Part model, mm, in its own coordinate system. A direction names the side the tool comes from. Give positions to 0.01 mm unless a question says otherwise; leave off trailing zeros. Write each loop counter-clockwise with the first axis right and the second up, starting at its lowest first coordinate (ties: lowest second). Pieces come first, ordered by that corner, then holes.
from build123d import *

# Parameters (mm, degrees)
SKETCH_1_R          = 1.680805835
SKETCH_1_R_2        = 0.406348663
SKETCH_1_R_3        = 0.591052601
SKETCH_1_R_4        = 0.609522995
SKETCH_1_R_5        = 0.664934176
SKETCH_1_R_6        = 1.662335441
SKETCH_1_R_7        = 1.6
EXTRUDE_2_DEPTH     = 1.5
SKETCH_2_W          = 5
SKETCH_2_H          = 30
EXTRUDE_3_DEPTH     = 5
SKETCH_3_W          = 46
SKETCH_3_H          = 35.259040571
EXTRUDE_4_DEPTH     = 1.2
SKETCH_4_W          = 16.562645757
SKETCH_4_H          = 20.676210758
EXTRUDE_5_DEPTH     = 15
SKETCH_5_W          = 14
SKETCH_5_H          = 12
CUT_EXTRUDE_1_DEPTH = 16
SKETCH_6_W          = 12.857554965
SKETCH_6_H          = 12.912362425
EXTRUDE_6_DEPTH     = 5
SKETCH_9_W          = 3.8
SKETCH_9_H          = 10.912362425
CUT_EXTRUDE_2_DEPTH = 11


with BuildPart() as part:
    # 草图1 → 凸台-拉伸2 (new body)
    with BuildSketch(Plane.XY):
        with BuildLine():
            Line((42.436427683, 56.053220537), (165.136427683, 56.053220537))
            ThreePointArc((165.136427683, 56.053220537), (167.867822265, 57.210483747), (168.936427683, 59.977767064))
            Line((168.936427683, 59.977767064), (168.936427683, 152.253220537))
            ThreePointArc((168.936427683, 152.253220537), (167.823433451, 154.940226305), (165.136427683, 156.053220537))
            Line((165.136427683, 156.053220537), (42.436427683, 156.053220537))
            ThreePointArc((42.436427683, 156.053220537), (39.961553949, 155.028094271), (38.936427683, 152.553220537))
            Line((38.936427683, 152.553220537), (38.936427683, 59.553220537))
            ThreePointArc((38.936427683, 59.553220537), (39.961553949, 57.078346802), (42.436427683, 56.053220537))
        make_face()
        with Locations((153.770781099, 129.383220537)):
            Circle(SKETCH_1_R, mode=Mode.SUBTRACT)
        with Locations((117.383571785, 118.473779489)):
            Circle(SKETCH_1_R_2, mode=Mode.SUBTRACT)
        with Locations((80.77524922, 90.287954645)):
            Circle(SKETCH_1_R_3, mode=Mode.SUBTRACT)
        with Locations((117.36509862, 90.269480326)):
            Circle(SKETCH_1_R_4, mode=Mode.SUBTRACT)
        with Locations((80.775251991, 118.436830852)):
            Circle(SKETCH_1_R_2, mode=Mode.SUBTRACT)
        with Locations((77.930808577, 120.563856588)):
            Circle(SKETCH_1_R_5, mode=Mode.SUBTRACT)
        with Locations((120.330808475, 120.56092691)):
            Circle(SKETCH_1_R_5, mode=Mode.SUBTRACT)
        with Locations((120.301889386, 88.163856588)):
            Circle(SKETCH_1_R_5, mode=Mode.SUBTRACT)
        with Locations((77.930808577, 88.163856588)):
            Circle(SKETCH_1_R_5, mode=Mode.SUBTRACT)
        with Locations((165.170781099, 59.633220537)):
            Circle(SKETCH_1_R_6, mode=Mode.SUBTRACT)
        with Locations((165.170781099, 152.133220537)):
            Circle(SKETCH_1_R, mode=Mode.SUBTRACT)
        with Locations((42.470781099, 152.483220537)):
            Circle(SKETCH_1_R, mode=Mode.SUBTRACT)
        with Locations((42.470781099, 59.283220537)):
            Circle(SKETCH_1_R, mode=Mode.SUBTRACT)
        with Locations(Location((153.770781099, 74.383220537, 0), (0, 0, 180))):
            Circle(SKETCH_1_R, mode=Mode.SUBTRACT)
        with Locations(Location((41.470781099, 74.383220537, 0), (0, 0, 180))):
            Circle(SKETCH_1_R_7, mode=Mode.SUBTRACT)
        with Locations((41.470781099, 129.383220537)):
            Circle(SKETCH_1_R_7, mode=Mode.SUBTRACT)
    extrude(amount=EXTRUDE_2_DEPTH)

    # 草图2 → 凸台-拉伸3 (add)
    with BuildSketch(Plane.XY.offset(1.5)):
        with Locations((80.750808475, 104.36092691)):
            Rectangle(SKETCH_2_W, SKETCH_2_H)
        with Locations((117.510808475, 104.36092691)):
            Rectangle(SKETCH_2_W, SKETCH_2_H)
    extrude(amount=EXTRUDE_3_DEPTH)

    # 草图3 → 凸台-拉伸4 (add)
    with BuildSketch(Plane.XY.offset(6.5)):
        with Locations((99.230808475, 104.360926909)):
            Rectangle(SKETCH_3_W, SKETCH_3_H)
    extrude(amount=EXTRUDE_4_DEPTH)

    # 草图4 → 凸台-拉伸5 (add)
    with BuildSketch(Plane.XY.offset(1.5)):
        with Locations((141.730083201, 145.715115158)):
            Rectangle(SKETCH_4_W, SKETCH_4_H)
    extrude(amount=EXTRUDE_5_DEPTH)

    # 草图5 → 切除-拉伸1 (cut)
    with BuildSketch(Plane(origin=(0, 156.053220537, 0), x_dir=(1, 0, 0), z_dir=(0, 1, 0))):
        with Locations((141.815149852, -7.784103515)):
            Rectangle(SKETCH_5_W, SKETCH_5_H)
    extrude(amount=-CUT_EXTRUDE_1_DEPTH, mode=Mode.SUBTRACT)

    # 草图6 → 凸台-拉伸6 (add)
    with BuildSketch(Plane.XY.offset(1.5)):
        with Locations((45.365205166, 85.403032826)):
            Rectangle(SKETCH_6_W, SKETCH_6_H)
    extrude(amount=EXTRUDE_6_DEPTH)

    # 草图9 → 切除-拉伸2 (cut)
    with BuildSketch(Plane.ZY.offset(-38.936427683)):
        with Locations((3.4, 85.403032826)):
            Rectangle(SKETCH_9_W, SKETCH_9_H)
    extrude(amount=-CUT_EXTRUDE_2_DEPTH, mode=Mode.SUBTRACT)


solid = part.part
1) Mould opens along X. For faces 6 (the flat face through (142, 135.377, 9)), 7 (the flat face through (148.815, 148, 8)), 8 (the cylindrical face through (167.84, 57.18, 0.74)) say: +X half, -X half, draft (parallel to the pull), parting line (faces both ways), or undercut.
Check result:
face 6: draft
face 7: undercut
face 8: +X half
2) Saw through at D-D (x = 48.5). Write the cut outline in (y, z), and give its area (3 significant figures).
Check result:
outline: (56.05, 0) - (156.05, 0) - (156.05, 1.5) - (91.86, 1.5) - (91.86, 6.5) - (78.95, 6.5) - (78.95, 1.5) - (56.05, 1.5) - close; hole (79.95, 1.5) - (90.86, 1.5) - (90.86, 5.3) - (79.95, 5.3) - close
area: 173 mm2
3) Saw through at C-C (x = 144). Write the cut outline in (y, z).
Check result:
outline: (56.05, 0) - (156.05, 0) - (156.05, 1.78) - (140.05, 1.78) - (140.05, 13.78) - (156.05, 13.78) - (156.05, 16.5) - (135.38, 16.5) - (135.38, 1.5) - (56.05, 1.5) - close
4) Flat gauge pins, fed straight in: P1, Ø2, axis at x = 117.5, y = 67.5, coming from the +Z side; P2, Ø1.5, axis at x = 42.5, z = 3.5, coming from the +Y side; P3, Ø8, axis at x = 82.5, y = 99.5, coming from the +Z side. Where does each tip first touch, or does it go through?
Check result:
P1: stops at z = 1.5
P2: stops at y = 91.86
P3: stops at z = 7.7
5) 3-axis set-ups, long thin cutter, end or side, ignore diameter. For faces 1 (the flat face through (81, 119.361, 4)), 2 (the flat face through (45, 91.859, 4)), 3 (the flat face through (142, 148, 13.784)), 4 (the flat face through (45, 78.947, 4)), 5 (the flat face through (44, 79.947, 3)): which of +Z, -Z, +X, -X, +Y, -Y reach the whole face in a straight line?
Check result:
face 1: +X, -X, +Y
face 2: +Z, -X, +Y
face 3: +Y
face 4: +Z, +X, -X, -Y
face 5: -X
6) Saw through at A-A (x = 113). Write the cut outline in (y, z), and give its area (3 significant figures).
Check result:
outline: (56.05, 0) - (156.05, 0) - (156.05, 1.5) - (56.05, 1.5) - close; (86.73, 6.5) - (121.99, 6.5) - (121.99, 7.7) - (86.73, 7.7) - close
area: 192 mm2
7) Drill centre lines: L1, parallel to X at y = 150, z = 8.25; L2, parallel to X at y = 102.5, z = 4.75; L3, parallel to Z at x = 163, y = 99.5. Where is each one in solid material? Low to high.
Check result:
L1: x = 133.45 to 134.82, 148.82 to 150.01
L2: x = 78.25 to 83.25, 115.01 to 120.01
L3: z = 0 to 1.5
8) Saw through at B-B (z = 10). Write the cut outline in (x, y).
Check result:
outline: (133.45, 135.38) - (150.01, 135.38) - (150.01, 156.05) - (148.82, 156.05) - (148.82, 140.05) - (134.82, 140.05) - (134.82, 156.05) - (133.45, 156.05) - close
